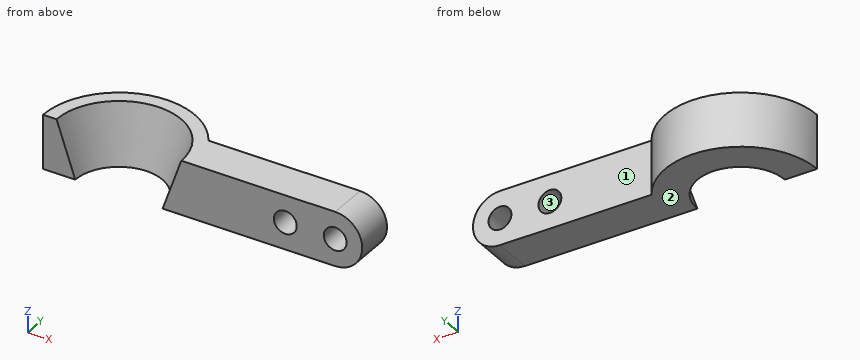
from build123d import *

# Parameters (mm, degrees)
F1_ANGLE = 180
F2_R     = 11
F3_DEPTH = 38


with BuildPart() as f1:
    # F0 (on Front) → F1 (revolve)
    with BuildSketch(Plane.XZ):
        Polygon((-73, 0), (-42, 0), (-60, 52), (-73, 52), align=None)
    revolve(axis=Axis((0, 0, 26.369863), (0, 0, -1)), revolution_arc=F1_ANGLE)

    # F2 (on Front) → F3 (join)
    with BuildSketch(Plane.XZ):
        with BuildLine():
            Line((60, 52), (60, 0))
            Line((60, 0), (208, 0))
            ThreePointArc((208, 0), (234, 26), (208, 52))
            Line((208, 52), (73, 52))
            Line((73, 52), (60, 52))
        make_face()
        with Locations((160, 26)):
            Circle(F2_R, mode=Mode.SUBTRACT)
        with Locations((208, 26)):
            Circle(F2_R, mode=Mode.SUBTRACT)
    extrude(amount=-F3_DEPTH)


solid = f1.part
Check sheet for the modelled part. Datum: model origin and axes. Units: mm. Face numbers are marked on the shaded views. Coordinates: 2 decimals unless noted, no trailing zeros. Write each loop counter-clockwise with the first axis right and the second up, starting at its lowest first coordinate (ties: lowest second). Pieces come first, ordered by that corner, then holes.
Item 1: Depth check by flat-ended pin: pin 1 Ø8 at (y, z) = (19.5, 21.5) entering from +X; pin 2 Ø1.5 at (y, z) = (16.5, 45.5) entering from +X; pin 3 Ø4 at (y, z) = (37, 44.5) entering from -X. Enter the tip coordinate at first touch or a pass-through.
Numbers:
pin 1: stops at x = 234
pin 2: stops at x = 226.01
pin 3: stops at x = -64.06
Item 2: Cross-section at C-C on y = 30. Count the separate pieces of the cut face and the enclosed holes in it, then the cut area to 3 significant figures.
Numbers:
separate pieces: 2
enclosed holes: 2
area: 10,300 mm2
Item 3: Scan lines: probe 1 along Z at (x, y) = (160, 19); probe 2 along Y at (x, z) = (122.5, 50); probe 3 along X at (y, z) = (39, 33.5). Record each from-to range of solid material in increasing order.
Numbers:
probe 1: z = 0 to 15, 37 to 52
probe 2: y = 0 to 38
probe 3: x = -61.71 to -36.76, 36.76 to 61.71
Item 4: Mould release check, pull along Z, two halves, no side actions. Record for the marked faces 1, 2 and 3: released by +Z, released by -Z, zero draft, split by the parting line, or undercut.
Numbers:
face 1: zero draft
face 2: released by -Z
face 3: undercut
Item 5: Cross-section at A-A on z = 26. Record the boundary of the cut face in (x, y), then the cut area to 3 significant figures.
Numbers:
outline: (-73, 0) - (-51, 0) arc R51 cw to (51, 0) - (149, 0) - (149, 38) - (62.33, 38) arc R73 ccw to start; (171, 0) - (197, 0) - (197, 38) - (171, 38) - close; (219, 0) - (234, 0) - (234, 38) - (219, 38) - close
area: 8,860 mm2
Item 6: Cross-section at B-B on x = 160. Record the boundary of the cut face in (y, z), then the cut area to 3 significant figures.
Numbers:
outline: (0, 0) - (38, 0) - (38, 15) - (0, 15) - close; (0, 37) - (38, 37) - (38, 52) - (0, 52) - close
area: 1,140 mm2
Item 7: Cross-section at D-D on x = 0. Record the boundary of the cut face in (y, z), then the cut area to 3 significant figures.
Numbers:
outline: (42, 0) - (73, 0) - (73, 52) - (60, 52) - close
area: 1,140 mm2
